```python
from build123d import *

# Parameters (mm, degrees)
EXTRUDE_1_DEPTH    = 60
CHAMFER3_SIZE2     = 11.912970931
CHAMFER3_SIZE      = 60
CHAMFER4_SIZE2     = 11.912970931
CHAMFER4_SIZE      = 60
CHAMFER5_SIZE2     = 9.519169095
CHAMFER5_SIZE      = 60
CUT_EXTRUDE1_DEPTH = 1279.275631979


with BuildPart() as part:
    # Эскиз1 → Бобышка-Вытянуть1 (new body)
    with BuildSketch(Plane.XY):
        Polygon((-849.589927609, 515.838957491), (787.506047005, 606.405063543), (281.615569427, -953.197537878), align=None)
    extrude(amount=EXTRUDE_1_DEPTH)

    # Chamfer3
    chamfer3_edges = [part.edges().sort_by_distance(p)[0] for p in [
        (-31.041940302, 561.122010517, 60),
    ]]
    chamfer3_side = [part.faces().sort_by_distance(p)[0] for p in [
        (-31.041940302, 561.122010517, 59.761740581),
    ]]
    chamfer(chamfer3_edges, length=CHAMFER3_SIZE - 0.0001, length2=CHAMFER3_SIZE2 - 0.0001, reference=chamfer3_side[0])  # a hair under: the kernel refuses the full size

    # Chamfer4
    chamfer4_edges = [part.edges().sort_by_distance(p)[0] for p in [
        (532.590398399, -179.470785737, 60),
    ]]
    chamfer4_side = [part.faces().sort_by_distance(p)[0] for p in [
        (532.590398399, -179.470785737, 59.761740581),
    ]]
    chamfer(chamfer4_edges, length=CHAMFER4_SIZE - 0.0001, length2=CHAMFER4_SIZE2 - 0.0001, reference=chamfer4_side[0])  # a hair under: the kernel refuses the full size

    # Chamfer5
    chamfer5_edges = [part.edges().sort_by_distance(p)[0] for p in [
        (-283.987179091, -218.679290193, 60),
    ]]
    chamfer5_side = [part.faces().sort_by_distance(p)[0] for p in [
        (-283.987179091, -218.679290193, 59.809616618),
    ]]
    chamfer(chamfer5_edges, length=CHAMFER5_SIZE - 0.0001, length2=CHAMFER5_SIZE2 - 0.0001, reference=chamfer5_side[0])  # a hair under: the kernel refuses the full size

    # Sketch1 → Cut-Extrude1 (cut, through all)
    with BuildSketch(Plane(origin=(0, 0, 0), x_dir=(-1, 0, 0), z_dir=(0, 0, -1))):
        Polygon((-534.560808216, -173.396237168), (31.041940302, 561.122010517), (-787.506047005, 606.405063543), align=None)
    extrude(amount=-CUT_EXTRUDE1_DEPTH, mode=Mode.SUBTRACT)


solid = part.part
```
Check sheet for the modelled part. Datum: model origin and axes. Units: mm. Round coordinates to 2 decimals unless told otherwise and drop trailing zeros. Write each loop counter-clockwise with the first axis right and the second up, starting at its lowest first coordinate (ties: lowest second). Pieces come first, ordered by that corner, then holes. Notation, with made-up numbers: M 80,27 L 95,27 A20 ccw 95,48 Z; hole C 7.5,23.25 d5. An arc over 180 degrees is marked long. Write item = value, one per line. Start each with the question number.
1. Release check for a two-part mould opening along X. For faces 1 (the flat face through (255.72, 188.72, 29.58)), 2 (the flat face through (-272.245, -226.018, 30.42)), 3 (the flat face through (6, -17, 0)) record: pulls with the +X half, pulls with the -X half, needs draft (parallel to the pull), parting line crosses it, or undercut.
2. Gauge pin test, flat ends, axial feed: pin 1 (5 mm diameter, centred on y = 198.5, z = 10.5, fed in from +X); pin 2 (6 mm diameter, centred on x = 147.5, z = 8, fed in from -Y); pin 3 (1 mm diameter, centred on y = -230.5, z = 25, fed in from +X). Record the tip position at first contact, or that the pin passes through.
3. Scan lines: line 1 (Y direction, x = 160.5, z = 45.5); line 2 (Y direction, x = -553.5, z = 54); line 3 (X direction, y = -299, z = 55.5). Record each from-to range of solid material in increasing order. Write a range as [from, to].
4. Section check C-C, the plane z = 50.5. Record the cut outline in (x, y).
Results found:
q1.face_1 = pulls with the +X half
q1.face_2 = pulls with the -X half
q1.face_3 = needs draft
q2.pin_1 = 250.11
q2.pin_2 = -780.92
q2.pin_3 = 511.01
q3.line_1 = [-784.08, 312.38]
q3.line_2 = [145.36, 521.48]
q3.line_3 = [-211.02, 482.23]
q4.outline = M -832.47,506.74 L 277.2,-934.33 L 527.14,-163.76 L -23.63,551.49 Z
